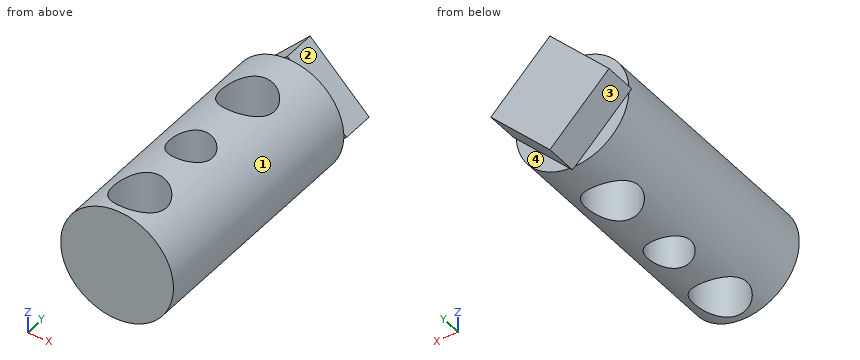
```python
from build123d import *

# Parameters (mm, degrees)
F0_R          = 6.75
F1_DEPTH      = 13
F1_DEPTH_BACK = 17
F2_R          = 3.175
F2_R_2        = 2.5796875
F3_DEPTH      = 6.751
F3_DEPTH_BACK = 6.751
F5_DEPTH      = 4


with BuildPart() as f1:
    # F0 (on Front) → F1 (new body, two sides)
    with BuildSketch(Plane.XZ) as f1_sk:
        Circle(F0_R)
    extrude(amount=-F1_DEPTH)
    extrude(f1_sk.sketch, amount=F1_DEPTH_BACK)

    # F2 (on Top) → F3 (cut, two sides)
    with BuildSketch(Plane.XY) as f3_sk:
        with Locations((0, 6)):
            Circle(F2_R)
        with Locations((0, -4)):
            Circle(F2_R_2)
        with Locations((0, -13)):
            Circle(F2_R)
    extrude(amount=-F3_DEPTH, mode=Mode.SUBTRACT)
    extrude(f3_sk.sketch, amount=F3_DEPTH_BACK, mode=Mode.SUBTRACT)

    # F4 (on face) → F5 (join)
    with BuildSketch(Plane(origin=(0, 13, 0), x_dir=(-1, 0, 0), z_dir=(0, 1, 0))):
        Polygon((-7.0710678119, 0), (0, -7.0710678119), (7.0710678119, 0), (0, 7.0710678119), align=None)
    extrude(amount=F5_DEPTH)


solid = f1.part
```
Geometry check sheet. Reference: the model listing, model coordinates, mm. Face numbers are marked on the shaded views. A direction names the side the tool comes from. Give positions to 0.01 mm unless a question says otherwise; leave off trailing zeros. Order: outer loops, then holes, each group sorted by start corner. A loop starts at its lowest first (then second) coordinate and runs counter-clockwise, first axis right, second up. Notation, with made-up numbers: (11.25, -4.75) - (26.25, -4.75) arc R15 cw to (26.25, 24.25) - close; hole circle Ø11 at (-6, 49.25). An arc over 180 degrees is marked (long way). Write item = value, one per line. Start each with the question number.
1) Access from +Z, -Z, +X, -X, +Y, -Y to the whole of each face (thin tool, end or side, straight path). Record for the marked faces 1, 2, 3 and 4.
2) Section check B-B (y = -4). Enter the section's corners in (x, z), then the cut area to 3 significant figures.
3) Section check C-C (x = -5). Enter the section's corners in (y, z).
4) Scan lines: L1, parallel to Y at x = 0, z = 3.75 (3 decimals); L2, parallel to X at y = -11, z = 4.25; L3, parallel to X at y = 6, z = 4.25 (3 decimals). Record each from-to range of solid material in increasing order.
5) Section check A-A (z = -2). Enter the section's corners in (x, y) (3 decimals), then the cut area to 3 significant figures.
6) Gauge pin test, flat ends, axial feed: pin 1 Ø8 at (x, y) = (-3, 8) entering from +Z; pin 2 Ø2 at (x, y) = (1, -1) entering from -Z; pin 3 Ø3 at (x, z) = (5, -3) entering from +Y; pin 4 Ø1 at (x, y) = (5, 7) entering from +Z. Record the tip position at first contact, or that the pin passes through.
7) Section check D-D (y = -7.5). Enter the section's corners in (x, z), then the cut area to 3 significant figures.
Geometry check:
q1.face_1 = -Y
q1.face_2 = +Z, +X, +Y
q1.face_3 = -Z, -X, +Y
q1.face_4 = -Z, +X, +Y
q2.outline = (-2.58, -6.24) - (-2.58, 6.24) arc R6.75 ccw to start; (2.58, -6.24) arc R6.75 ccw to (2.58, 6.24) - close
q2.area = 75.2 mm2
q3.outline = (-17, -4.53) - (13, -4.53) - (13, -2.07) - (17, -2.07) - (17, 2.07) - (13, 2.07) - (13, 4.53) - (-17, 4.53) - close
q4.L1 = -17 to -16.175, -9.825 to -6.58, -1.42 to 2.825, 9.175 to 17
q4.L2 = -5.24 to -2.47, 2.47 to 5.24
q4.L3 = -5.244 to -3.175, 3.175 to 5.244
q5.outline = (-6.447, -17) - (6.447, -17) - (6.447, 13) - (5.071, 13) - (5.071, 17) - (-5.071, 17) - (-5.071, 13) - (-6.447, 13) - close; hole circle Ø6.35 at (0, -13); hole circle Ø6.35 at (0, 6); hole circle Ø5.159 at (0, -4)
q5.area = 343 mm2
q6.pin_1 = 6.75
q6.pin_2 = -6.75
q6.pin_3 = 17
q6.pin_4 = 5.03
q7.outline = circle Ø13.5 at (0, 0)
q7.area = 143 mm2
